from build123d import *
from build123d.topology import SkipClean

# Parameters (mm, degrees)
SKETCH1_R         = 19.05
SKETCH1_R_2       = 17.399
EXTRUDE1_DEPTH    = 63.5
EXTRUDE2_START    = 12.7
SKETCH2_R         = 34.671
SKETCH2_R_2       = 17.399
EXTRUDE2_DEPTH    = 12.7
SKETCH3_R         = 101.219
SKETCH3_R_2       = 17.399
EXTRUDE3_DEPTH    = 22.352
EXTRUDE4_REACH    = 175.79
SKETCH4_R         = 4.2164
CIRPATTERN1_COUNT = 20
EXTRUDE5_REACH    = 175.79
SKETCH6_R         = 3.3655
CIRPATTERN2_COUNT = 6


with BuildPart() as part:
    # Sketch1 → Extrude1 (new body)
    with BuildSketch(Plane(origin=(0, 0, 0), x_dir=(1, 0, 0), z_dir=(0, 1, 0))):
        with Locations(Location((0, 0, 0), (0, 0, 270))):
            Circle(SKETCH1_R)
        with Locations(Location((0, 0, 0), (0, 0, 270))):
            Circle(SKETCH1_R_2, mode=Mode.SUBTRACT)
    extrude(amount=EXTRUDE1_DEPTH)

    # Sketch2 → Extrude2 (add)
    with SkipClean():  # the faces are left unmerged after this step: merging them gives an invalid solid
        with BuildSketch(Plane.XZ.offset(EXTRUDE2_START)):
            with Locations(Location((0, 0, 0), (0, 0, 270))):
                Circle(SKETCH2_R)
            with Locations(Location((0, 0, 0), (0, 0, 270))):
                Circle(SKETCH2_R_2, mode=Mode.SUBTRACT)
        extrude(amount=-EXTRUDE2_DEPTH)

    # Sketch3 → Extrude3 (add)
    with BuildSketch(Plane(origin=(0, 63.5, 0), x_dir=(1, 0, 0), z_dir=(0, 1, 0))):
        with Locations(Location((0, 0, 0), (0, 0, 270))):
            Circle(SKETCH3_R)
        with Locations(Location((0, 0, 0), (0, 0, 90))):
            Circle(SKETCH3_R_2, mode=Mode.SUBTRACT)
    extrude(amount=EXTRUDE3_DEPTH)

    # Sketch4 → Extrude4 (cut, up to next)
    with BuildSketch(Plane(origin=(0, 85.852, 0), x_dir=(1, 0, 0), z_dir=(0, 1, 0)), mode=Mode.PRIVATE) as extrude4_sk1:
        with Locations(Location((0, 90.5256, 0), (0, 0, 270))):
            Circle(SKETCH4_R)
    extrude4_tool1 = extrude(extrude4_sk1.sketch, amount=-EXTRUDE4_REACH, mode=Mode.PRIVATE) & part.part
    extrude4 = extrude4_tool1.solids().sort_by_distance((0, 85.852, -90.5256))[0]
    add(extrude4, mode=Mode.SUBTRACT)

    # CirPattern1: Extrude4 ×20 about axis
    cirpattern1_axis = Axis((0, 0, 0), (0, 1, 0))
    for i in range(1, CIRPATTERN1_COUNT):
        add(extrude4.rotate(cirpattern1_axis, i * 360 / CIRPATTERN1_COUNT), mode=Mode.SUBTRACT)

    # Sketch6 → Extrude5 (cut, up to next)
    with BuildSketch(Plane.XZ.offset(12.7), mode=Mode.PRIVATE) as extrude5_sk1:
        with Locations(Location((0, 29.3624, 0), (0, 0, 270))):
            Circle(SKETCH6_R)
    extrude5_tool1 = extrude(extrude5_sk1.sketch, amount=-EXTRUDE5_REACH, mode=Mode.PRIVATE) & part.part
    extrude5 = extrude5_tool1.solids().sort_by_distance((0, -12.7, 29.3624))[0]
    add(extrude5, mode=Mode.SUBTRACT)

    # CirPattern2: Extrude5 ×6 about axis
    cirpattern2_axis = Axis((0, 0, 0), (0, 1, 0))
    for i in range(1, CIRPATTERN2_COUNT):
        add(extrude5.rotate(cirpattern2_axis, i * 360 / CIRPATTERN2_COUNT), mode=Mode.SUBTRACT)


solid = part.part
CAD build for the part. Positions are in the model's coordinates, mm. A direction names the side the tool comes from. Round coordinates to 2 decimals unless told otherwise and drop trailing zeros. Order: outer loops, then holes, each group sorted by start corner. A loop starts at its lowest first (then second) coordinate and runs counter-clockwise, first axis right, second up. Notation, with made-up numbers: (-13.5, 53) - (26.5, 53) arc R21 ccw to (26.5, 72) - close; hole circle Ø10 at (32, 50). An arc over 180 degrees is marked (long way). Return JSON: item names as keys, results as strings.
(1) Pin check, flat tips, straight feed: pin 1 Ø13.5 at (x, z) = (86.09, 27.97) entering from +Y; pin 2 Ø3 at (x, z) = (-51.5, 49) entering from -Y; pin 3 Ø1.5 at (y, z) = (69.5, -12.5) entering from -X. Stop position of each tip, or through.
Answer key:
{"pin 1": "stops at y = 85.85", "pin 2": "stops at y = 63.5", "pin 3": "stops at x = -100.53"}
(2) Cut at A-A (z = 0). Give the cut face in (x, y), then the cut area to 3 significant figures.
Answer key:
{"outline": "(-101.22, 63.5) - (-94.74, 63.5) - (-94.74, 85.85) - (-101.22, 85.85) - close; (-86.31, 63.5) - (-19.05, 63.5) - (-19.05, 0) - (-34.67, 0) - (-34.67, -12.7) - (-17.4, -12.7) - (-17.4, 85.85) - (-86.31, 85.85) - close; (17.4, -12.7) - (34.67, -12.7) - (34.67, 0) - (19.05, 0) - (19.05, 63.5) - (86.31, 63.5) - (86.31, 85.85) - (17.4, 85.85) - close; (94.74, 63.5) - (101.22, 63.5) - (101.22, 85.85) - (94.74, 85.85) - close", "area": "4,020 mm^2"}
(3) Wall check: probe 1 along Z at (x, y) = (-57, 72); probe 2 along Z at (x, y) = (72, 75); probe 3 along Y at (x, z) = (-16.5, -13). Give the ranges that are in metal, low to high. Write a range as from..to.
Answer key:
{"probe 1": "z = -83.64..-75.08, -71.39..71.39, 75.08..83.64", "probe 2": "z = -71.14..-57.24, -49.18..49.18, 57.24..71.14", "probe 3": "y = -12.7..0, 63.5..85.85"}
(4) Tool access for faces 4 (the face through (-55.836, 74.832, 76.536)), 5 (the face through (22.59, -6.44, 16.49)): list every direction of +Z, -Z, +X, -X, +Y, -Y with a clear straight run to the whole face (end or side of a thin tool).
Answer key:
{"face 4": "+Y, -Y", "face 5": "-Y"}
(5) Pull direction Y, two halves, no side cores. Call faces 1 (the face through (-21, 85.852, -1)), 2 (the face through (-11.59, 31.31, -15.12)), 3 (the face through (-26.22, 74.83, -89.93)): +Y half, -Y half, draft (parallel to the pull), parting line (faces both ways), or undercut.
Answer key:
{"face 1": "+Y half", "face 2": "undercut", "face 3": "draft"}
(6) Cut at D-D (y = 59). Give the cut face in (x, z), then the cut area to 3 significant figures.
Answer key:
{"outline": "circle Ø38.1 at (0, 0); hole circle Ø34.8 at (0, 0)", "area": "189 mm^2"}
(7) Cut at B-B (x = 0). State how many separate pieces and enclosed holes the cut face has, then the cut area to 3 significant figures.
Answer key:
{"separate pieces": "6", "enclosed holes": "0", "area": "3,850 mm^2"}
